```python
from build123d import *

# Parameters (mm, degrees)
F0_R     = 92.075
F0_R_2   = 20.75
F1_DEPTH = 25.4
F2_R     = 10
F3_DEPTH = 25.4
F5_D     = 10.71626
F6_SIZE  = 1.524


with BuildPart() as f1:
    # F0 (on Front) → F1 (new body)
    with BuildSketch(Plane.XZ):
        Circle(F0_R)
        Circle(F0_R_2, mode=Mode.SUBTRACT)
    extrude(amount=-F1_DEPTH)

    # F2 (on face) → F3 (cut)
    with BuildSketch(Plane.XZ):
        with Locations((-57.3634247583, 20)):
            Circle(F2_R)
        with Locations((-20, 57.3634247583)):
            Circle(F2_R)
        with Locations((57.3634247583, -20)):
            Circle(F2_R)
        with Locations((20, -57.3634247583)):
            Circle(F2_R)
    extrude(amount=-F3_DEPTH, mode=Mode.SUBTRACT)

    # F5 (through all)
    with Locations(Plane.XZ):
        with Locations((-35.9210244843, 35.9210244843), (35.9210244843, 35.9210244843), (35.9210244843, -35.9210244843), (-35.9210244843, -35.9210244843)):
            Hole(F5_D / 2)

    # F6
    f6_edges = [f1.edges().sort_by_distance(p)[0] for p in [
        (92.075, 12.7, 0),
        (-92.075, 0, 0),
        (-92.075, 25.4, 0),
    ]]
    chamfer(f6_edges, length=F6_SIZE)


solid = f1.part
```
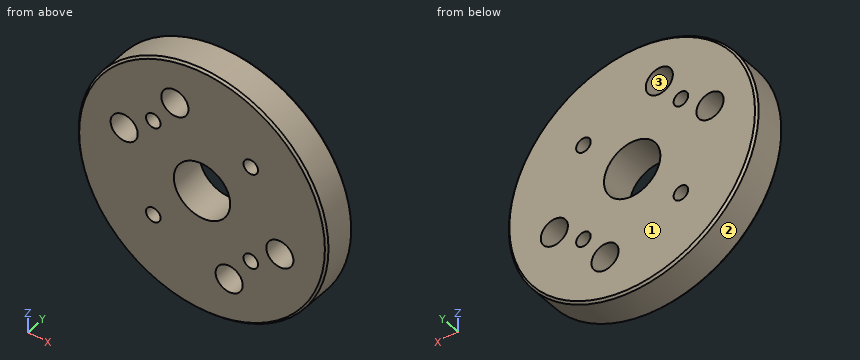
Can you work these out from the model? Positions are in its coordinate system, mm. Face numbers are marked on the shaded views. Round coordinates to 2 decimals unless told otherwise and drop trailing zeros. Loops run counter-clockwise (first coordinate to the right, second up) from the corner with the lowest first, then second, coordinate; pieces in that order, holes last. Notation, with made-up numbers: (-30.75, -38) -> (-4.75, -38) arc R19 cw to (-4.75, -8) -> close; hole circle Ø1 at (73, -25.5). An arc over 180 degrees is marked (long way). Answer in a Markdown table with one row per item.
Item 1: Suppose I cut it at C-C, the plane y = 4.25. Give the number of separate pieces and of enclosed holes in the cut face, plus the area to 3 significant figures.
Answer block:
| item | result |
|---|---|
| separate pieces | 1 |
| enclosed holes | 9 |
| area | 23,700 mm² |
Item 2: Suppose I cut it at B-B, the plane x = 0. List the corners of the cut face in (y, z) for me (3 decimals), plus the area to 3 significant figures.
Answer block:
| item | result |
|---|---|
| outline | (0, -90.551) -> (1.524, -92.075) -> (23.876, -92.075) -> (25.4, -90.551) -> (25.4, -20.75) -> (0, -20.75) -> close; (0, 20.75) -> (25.4, 20.75) -> (25.4, 90.551) -> (23.876, 92.075) -> (1.524, 92.075) -> (0, 90.551) -> close |
| area | 3,620 mm² |
Item 3: We'd pull the mould along X, two halves only. Please class the marked faces 1, 2 and 3: released by +X, released by -X, zero draft, split by the parting line, or undercut.
Answer block:
| item | result |
|---|---|
| face 1 | zero draft |
| face 2 | split by the parting line |
| face 3 | undercut |
Item 4: Suppose I cut it at A-A, the plane z = 0. List the corners of the cut face in (x, y) for me (3 decimals), plus the area to 3 significant figures.
Answer block:
| item | result |
|---|---|
| outline | (-92.075, 1.524) -> (-90.551, 0) -> (-20.75, 0) -> (-20.75, 25.4) -> (-90.551, 25.4) -> (-92.075, 23.876) -> close; (20.75, 0) -> (90.551, 0) -> (92.075, 1.524) -> (92.075, 23.876) -> (90.551, 25.4) -> (20.75, 25.4) -> close |
| area | 3,620 mm² |
Item 5: Will these pins go through, and if not, where does the flat tip stop? P1, Ø16, axis at x = 57.36, z = -20, coming from the -Y side; P2, Ø17, axis at x = 35.92, z = 35.92, coming from the +Y side; P3, Ø5, axis at y = 22, z = 39.5, coming from the +X side; P4, Ø2, axis at x = -8, y = 10.5, coming from the -Z side.
Answer block:
| item | result |
|---|---|
| P1 | through |
| P2 | y = 25.4 |
| P3 | x = 84.31 |
| P4 | z = -91.81 |
Item 6: If I drill on probe 1 along Z at (x, y) = (-17.5, 24); probe 2 along Z at (x, y) = (-17, 21); probe 3 along X at (y, z) = (2, -13.5), over which ranges is the centre line in solid material (lowest first)?
Answer block:
| item | result |
|---|---|
| probe 1 | -90.27 to -11.15, 11.15 to 47.68, 67.05 to 90.27 |
| probe 2 | -90.49 to -11.9, 11.9 to 47.82, 66.9 to 90.49 |
| probe 3 | -91.08 to -15.76, 15.76 to 49.76, 64.96 to 91.08 |
